Check sheet for the modelled part. Datum: model origin and axes. Units: mm. Round coordinates to 2 decimals unless told otherwise and drop trailing zeros. One line per item, written item: value.
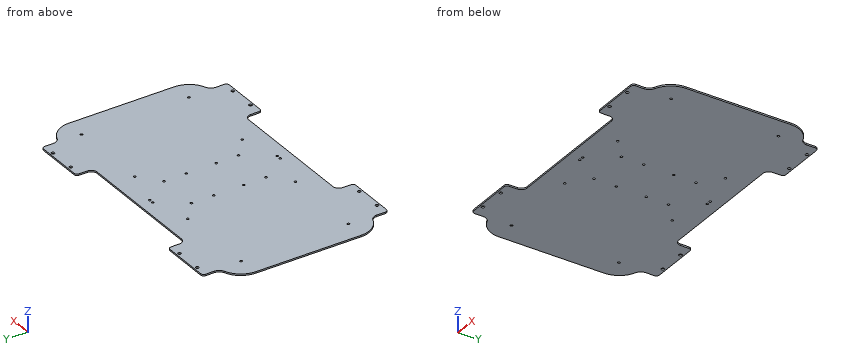
from build123d import *

# Parameters (mm, degrees)
SKETCH1_R           = 2.05
SKETCH1_R_2         = 1.55
BOSS_EXTRUDE1_DEPTH = 2
FILLET_1_R          = 10
FILLET_2_R          = 3
EXTRUDE_1_DEPTH     = 2
CUT_EXTRUDE_1_DEPTH = 10
FILLET_3_R          = 4
SKETCH5_R           = 1.55
CUT_EXTRUDE1_DEPTH  = 10


with BuildPart() as part:
    # Sketch1 → Boss-Extrude1 (new body)
    with BuildSketch(Plane.XY):
        Polygon((-89.5, -124.5), (-89.5, -101.5), (89.5, -101.5), (89.5, -124.5), (167.5, -124.5), (167.5, 124.5), (89.5, 124.5), (89.5, 101.5), (-89.5, 101.5), (-89.5, 124.5), (-167.5, 124.5), (-167.5, -124.5), align=None)
        with Locations((-146.5, -120.5)):
            Circle(SKETCH1_R, mode=Mode.SUBTRACT)
        with Locations((-110.5, -120.5)):
            Circle(SKETCH1_R, mode=Mode.SUBTRACT)
        with Locations((110.5, -120.5)):
            Circle(SKETCH1_R, mode=Mode.SUBTRACT)
        with Locations((146.5, -120.5)):
            Circle(SKETCH1_R, mode=Mode.SUBTRACT)
        with Locations((110.5, 120.5)):
            Circle(SKETCH1_R, mode=Mode.SUBTRACT)
        with Locations((146.5, 120.5)):
            Circle(SKETCH1_R, mode=Mode.SUBTRACT)
        with Locations((-110.5, 120.5)):
            Circle(SKETCH1_R, mode=Mode.SUBTRACT)
        with Locations((-146.5, 120.5)):
            Circle(SKETCH1_R, mode=Mode.SUBTRACT)
        with Locations((-28, -50)):
            Circle(SKETCH1_R_2, mode=Mode.SUBTRACT)
        with Locations((-28, -20)):
            Circle(SKETCH1_R_2, mode=Mode.SUBTRACT)
        with Locations((-28, 20)):
            Circle(SKETCH1_R_2, mode=Mode.SUBTRACT)
        with Locations((-28, 50)):
            Circle(SKETCH1_R_2, mode=Mode.SUBTRACT)
        with Locations((28, 50)):
            Circle(SKETCH1_R_2, mode=Mode.SUBTRACT)
        with Locations((28, 20)):
            Circle(SKETCH1_R_2, mode=Mode.SUBTRACT)
        with Locations((28, -20)):
            Circle(SKETCH1_R_2, mode=Mode.SUBTRACT)
        with Locations((28, -50)):
            Circle(SKETCH1_R_2, mode=Mode.SUBTRACT)
        with Locations((-162, -72)):
            Circle(SKETCH1_R_2, mode=Mode.SUBTRACT)
        with Locations((-54, -72)):
            Circle(SKETCH1_R_2, mode=Mode.SUBTRACT)
        with Locations((-162, 72)):
            Circle(SKETCH1_R_2, mode=Mode.SUBTRACT)
        with Locations((-54, 72)):
            Circle(SKETCH1_R_2, mode=Mode.SUBTRACT)
        with Locations((162, 72)):
            Circle(SKETCH1_R_2, mode=Mode.SUBTRACT)
        with Locations((54, 72)):
            Circle(SKETCH1_R_2, mode=Mode.SUBTRACT)
        with Locations((162, -72)):
            Circle(SKETCH1_R_2, mode=Mode.SUBTRACT)
        with Locations((54, -72)):
            Circle(SKETCH1_R_2, mode=Mode.SUBTRACT)
    extrude(amount=BOSS_EXTRUDE1_DEPTH)

    # 圆角1
    fillet_1_edges = [part.edges().sort_by_distance(p)[0] for p in [
        (-89.5, 101.5, 1),
        (89.5, 101.5, 1),
        (89.5, -101.5, 1),
        (-89.5, -101.5, 1),
    ]]
    fillet(fillet_1_edges, radius=FILLET_1_R)

    # 圆角2
    fillet_2_edges = [part.edges().sort_by_distance(p)[0] for p in [
        (89.5, 124.5, 1),
        (167.5, 124.5, 1),
        (167.5, -124.5, 1),
        (89.5, -124.5, 1),
        (-89.5, -124.5, 1),
        (-167.5, -124.5, 1),
        (-167.5, 124.5, 1),
        (-89.5, 124.5, 1),
    ]]
    fillet(fillet_2_edges, radius=FILLET_2_R)

    # 草图1 → 凸台-拉伸1 (add)
    with BuildSketch(Plane.XY.offset(2)):
        with BuildLine():
            Line((189.997376171, 0), (189.999999808, 70.585935638))
            ThreePointArc((189.999999808, 70.585935638), (184.491557968, 88.202366102), (169.927835286, 99.541657768))
            ThreePointArc((169.927835286, 99.541657768), (167.242378396, 101.21624095), (165.416431352, 103.801163566))
            Line((165.416431352, 103.801163566), (165.416428605, 0))
            Line((165.416428605, 0), (165.416431352, -103.801163566))
            ThreePointArc((165.416431352, -103.801163566), (167.242378396, -101.21624095), (169.927835286, -99.541657768))
            ThreePointArc((169.927835286, -99.541657768), (184.491557968, -88.202366102), (189.999999808, -70.585935638))
            Line((189.999999808, -70.585935638), (189.997376171, 0))
        make_face()
        with BuildLine():
            Line((-165.416431352, 103.801163566), (-165.416428605, 0))
            Line((-165.416428605, 0), (-165.416431352, -103.801163566))
            ThreePointArc((-165.416431352, -103.801163566), (-167.242378396, -101.21624095), (-169.927835286, -99.541657768))
            ThreePointArc((-169.927835286, -99.541657768), (-184.491557968, -88.202366102), (-189.999999808, -70.585935638))
            Line((-189.999999808, -70.585935638), (-189.997376171, 0))
            Line((-189.997376171, 0), (-189.999999808, 70.585935638))
            ThreePointArc((-189.999999808, 70.585935638), (-184.491557968, 88.202366102), (-169.927835286, 99.541657768))
            ThreePointArc((-169.927835286, 99.541657768), (-167.242378396, 101.21624095), (-165.416431352, 103.801163566))
        make_face()
    extrude(amount=-EXTRUDE_1_DEPTH)

    # 草图2 → 切除-拉伸1 (cut)
    with BuildSketch(Plane(origin=(0, 0, 0), x_dir=(-1, 0, 0), z_dir=(0, 0, -1))):
        with BuildLine():
            Line((-163.5, 108.882062038), (-163.5, 125.12763211))
            Line((-163.5, 125.12763211), (-195.489977478, 125.12763211))
            Line((-195.489977478, 125.12763211), (-189.999999808, 70.585935638))
            ThreePointArc((-189.999999808, 70.585935638), (-184.506224613, 88.181189445), (-169.976064889, 99.523542853))
            ThreePointArc((-169.976064889, 99.523542853), (-165.276881641, 103.191690833), (-163.5, 108.882062038))
        make_face()
        with BuildLine():
            Line((-60.806736633, 101.5), (-85.5, 101.5))
            ThreePointArc((-85.5, 101.5), (-91.156854249, 103.843145751), (-93.5, 109.5))
            Line((-93.5, 109.5), (-93.5, 125.12763211))
            Line((-93.5, 125.12763211), (-60.806736633, 125.12763211))
            Line((-60.806736633, 125.12763211), (-60.806736633, 101.5))
        make_face()
        with BuildLine():
            Line((60.806736633, 125.12763211), (60.806736633, 101.5))
            Line((60.806736633, 101.5), (85.5, 101.5))
            ThreePointArc((85.5, 101.5), (91.156854249, 103.843145751), (93.5, 109.5))
            Line((93.5, 109.5), (93.5, 125.12763211))
            Line((93.5, 125.12763211), (60.806736633, 125.12763211))
        make_face()
        with BuildLine():
            Line((195.489977478, 125.12763211), (189.999999808, 70.585935638))
            ThreePointArc((189.999999808, 70.585935638), (184.506224613, 88.181189445), (169.976064889, 99.523542853))
            ThreePointArc((169.976064889, 99.523542853), (165.276881641, 103.191690833), (163.5, 108.882062038))
            Line((163.5, 108.882062038), (163.5, 125.12763211))
            Line((163.5, 125.12763211), (195.489977478, 125.12763211))
        make_face()
        with BuildLine():
            Line((163.5, -108.882062038), (163.5, -125.12763211))
            Line((163.5, -125.12763211), (195.489977478, -125.12763211))
            Line((195.489977478, -125.12763211), (189.999999808, -70.585935638))
            ThreePointArc((189.999999808, -70.585935638), (184.506224613, -88.181189445), (169.976064889, -99.523542853))
            ThreePointArc((169.976064889, -99.523542853), (165.276881641, -103.191690833), (163.5, -108.882062038))
        make_face()
        with BuildLine():
            Line((60.806736633, -101.5), (85.5, -101.5))
            ThreePointArc((85.5, -101.5), (91.156854249, -103.843145751), (93.5, -109.5))
            Line((93.5, -109.5), (93.5, -125.12763211))
            Line((93.5, -125.12763211), (60.806736633, -125.12763211))
            Line((60.806736633, -125.12763211), (60.806736633, -101.5))
        make_face()
        with BuildLine():
            Line((-60.806736633, -125.12763211), (-60.806736633, -101.5))
            Line((-60.806736633, -101.5), (-85.5, -101.5))
            ThreePointArc((-85.5, -101.5), (-91.156854249, -103.843145751), (-93.5, -109.5))
            Line((-93.5, -109.5), (-93.5, -125.12763211))
            Line((-93.5, -125.12763211), (-60.806736633, -125.12763211))
        make_face()
        with BuildLine():
            Line((-195.489977478, -125.12763211), (-189.999999808, -70.585935638))
            ThreePointArc((-189.999999808, -70.585935638), (-184.506224613, -88.181189445), (-169.976064889, -99.523542853))
            ThreePointArc((-169.976064889, -99.523542853), (-165.276881641, -103.191690833), (-163.5, -108.882062038))
            Line((-163.5, -108.882062038), (-163.5, -125.12763211))
            Line((-163.5, -125.12763211), (-195.489977478, -125.12763211))
        make_face()
    extrude(amount=-CUT_EXTRUDE_1_DEPTH, mode=Mode.SUBTRACT)

    # 圆角3
    fillet_3_edges = [part.edges().sort_by_distance(p)[0] for p in [
        (93.5, 124.5, 1),
        (-93.5, 124.5, 1),
        (-163.5, 124.5, 1),
        (-163.5, -124.5, 1),
        (-93.5, -124.5, 1),
        (93.5, -124.5, 1),
        (163.5, -124.5, 1),
        (163.5, 124.5, 1),
    ]]
    fillet(fillet_3_edges, radius=FILLET_3_R)

    # Sketch5 → Cut-Extrude1 (cut)
    with BuildSketch(Plane(origin=(0, 0, 0), x_dir=(-1, 0, 0), z_dir=(0, 0, -1))):
        with Locations((3, 85.5)):
            Circle(SKETCH5_R)
        with Locations((-3, 85.5)):
            Circle(SKETCH5_R)
        with Locations((-3, -85.5)):
            Circle(SKETCH5_R)
        with Locations((3, -85.5)):
            Circle(SKETCH5_R)
    extrude(amount=-CUT_EXTRUDE1_DEPTH, mode=Mode.SUBTRACT)


solid = part.part
Item 1: Material ranges on line 1 along Y through (x, z) = (-3, 1.5); line 2 along X through (y, z) = (72, 1.45); line 3 along Y through (x, z) = (-110.5, 1.2), recorded low to high.
Result set:
line 1: -101.5 to -87.05, -83.95 to 83.95, 87.05 to 101.5
line 2: -189.97 to -163.55, -160.45 to -55.55, -52.45 to 52.45, 55.55 to 160.45, 163.55 to 189.97
line 3: -124.5 to -122.55, -118.45 to 118.45, 122.55 to 124.5
Item 2: Depth check by flat-ended pin: pin 1 (2.5 mm diameter, centred on x = -3, y = 85.5, fed in from +Z); pin 2 (1 mm diameter, centred on y = -115, z = 0.5, fed in from +X); pin 3 (1 mm diameter, centred on y = 8.5, z = 1, fed in from +X); pin 4 (1 mm diameter, centred on y = 113.5, z = 1.5, fed in from -X). Enter the tip coordinate at first touch or a pass-through.
Result set:
pin 1: through
pin 2: x = 163.5
pin 3: x = 190
pin 4: x = -163.5
Item 3: Sectioned sample at A-A (z = 0.5). State how many separate pieces and enclosed holes the cut face has, then the cut area to 3 significant figures.
Result set:
separate pieces: 1
enclosed holes: 28
area: 82,600 mm^2
